The model under review builds one solid part; all positions refer to its coordinate system, in mm. A direction names the side the tool comes from. Give positions to 0.01 mm unless a question says otherwise; leave off trailing zeros. Order: outer loops, then holes, each group sorted by start corner. A loop starts at its lowest first (then second) coordinate and runs counter-clockwise, first axis right, second up. Notation, with made-up numbers: (23, -11) - (74, -11) arc R21 ccw to (74, 9) - close; hole circle Ø8 at (-38.75, -26.75). An arc over 180 degrees is marked (long way). Use CSV: the item, a comma, the result in double quotes.
```python
from build123d import *

# Parameters (mm, degrees)
F1_DEPTH    = 8
F2_R        = 1.5
F3_DEPTH    = 7.001
F4_T4_DEPTH = 8
F4_S5_R     = 1.5
F4_T6_DEPTH = 6
F5_R        = 1
F6_R        = 1
F7_R        = 3
F8_DEPTH    = 3


# Not quite as in the source:
# - a fillet or chamfer that OpenCascade refuses, or shapes differently, is made with other operations: its cross-section is extruded or revolved along the edge and cut away or added


with BuildPart() as f1:
    # F0 (on Front) → F1 (new body)
    with BuildSketch(Plane.XZ):
        Polygon((5.1, 5.1), (5.1, -5.1), (-5.1, -5.1), (-5.1, 5.1), (-5.1, 8.1), (-5.1, 17.1), (-8.1, 17.1), (-8.1, 8.1), (-8.1, -8.1), (8.1, -8.1), (8.1, 8.1), (-1.1, 8.1), (-1.1, 17.1), (-4.1, 17.1), (-4.1, 8.1), (-4.1, 5.1), align=None)
    extrude(amount=F1_DEPTH)

    # F2 (on face) → F3 (cut, through all)
    with BuildSketch(Plane.YZ.offset(-1.1)):
        with Locations((-5, 11)):
            Circle(F2_R)
    extrude(amount=-F3_DEPTH, mode=Mode.SUBTRACT)

    # F4: chamfer of 3 on 1 edges, made by hand


with BuildPart() as f4_tool2:
    # F4_s3 → F4_t4 (new body)
    with BuildSketch(Plane.XZ):
        Polygon((1.9, 8.1), (-1.1, 11.1), (-1.1, 8.1), align=None)
    extrude(amount=F4_T4_DEPTH)

    # F4_s5 → F4_t6 (cut, symmetric)
    with BuildSketch(Plane.YZ.offset(0.4)):
        with Locations((-5, 11)):
            Circle(F4_S5_R)
    extrude(amount=F4_T6_DEPTH, both=True, mode=Mode.SUBTRACT)


with BuildPart() as f1_1:
    add(f1.part)

    # F4_t1: union F4_tool2
    add(f4_tool2.part)

    # F5
    f5_edges = [f1_1.edges().sort_by_distance(p)[0] for p in [
        (8.1, -4, -8.1),
        (8.1, -4, 8.1),
        (8.1, 0, 0),
        (8.1, -8, 0),
        (-8.1, -4, -8.1),
        (0, 0, -8.1),
        (0, -8, -8.1),
        (-8.1, -4, 17.1),
        (-8.1, 0, 4.5),
        (-8.1, -8, 4.5),
        (-1.1, -4, 17.1),
        (-1.1, 0, 14.1),
        (-1.1, -8, 14.1),
    ]]
    fillet(f5_edges, radius=F5_R)

    # F6
    f6_edges = [f1_1.edges().sort_by_distance(p)[0] for p in [
        (0.4, 0, 9.6),
        (0.4, -8, 9.6),
    ]]
    fillet(f6_edges, radius=F6_R)

    # F7 (on face) → F8 (cut)
    with BuildSketch(Plane.YZ.offset(-1.1)):
        with Locations((-5, 11)):
            Circle(F7_R)
    extrude(amount=F8_DEPTH, mode=Mode.SUBTRACT)


solid = f1_1.part
```
Item 1: Mouldability with a two-part tool opening along X and no side actions: class faces 1 (the face through (7.799, -0.285, 0.606)), 2 (the face through (-5.1, -4, 6)), 3 (the face through (-6.6, -6.2, 10.1)) as pulls with the +X half, pulls with the -X half, needs draft (parallel to the pull), parting line crosses it, or undercut.
Results list:
face 1,"pulls with the +X half"
face 2,"undercut"
face 3,"needs draft"
Item 2: Wall thickness on L1, parallel to Z at x = -2.6, y = -5; L2, parallel to Y at x = -2.6, z = 11; L3, parallel to X at y = -5.5, z = -2.5: over which ranges is each line inside the solid? List them lowest first.
Results list:
L1,"z = -8.1 to -5.1, 5.1 to 9.5, 12.5 to 17.1"
L2,"y = -8 to -6.5, -3.5 to 0"
L3,"x = -8.1 to -5.1, 5.1 to 8.1"
Item 3: Take a section at B-B, the plane z = 14.25. Give the boundary of the cut face in (x, y).
Results list:
outline,"(-8.1, -7) arc R1 ccw to (-7.1, -8) - (-5.1, -8) - (-5.1, 0) - (-7.1, 0) arc R1 ccw to (-8.1, -1) - close; (-4.1, -8) - (-2.1, -8) arc R1 ccw to (-1.1, -7) - (-1.1, -1) arc R1 ccw to (-2.1, 0) - (-4.1, 0) - close"
Item 4: Take a section at C-C, the plane y = -5. Give the boundary of the cut face in (x, z), and give its area (3 significant figures).
Results list:
outline,"(-8.1, -7.1) arc R1 ccw to (-7.1, -8.1) - (7.1, -8.1) arc R1 ccw to (8.1, -7.1) - (8.1, 7.1) arc R1 ccw to (7.1, 8.1) - (1.9, 8.1) - (1.9, 8) - (-1.1, 8) - (-1.1, 9.5) - (-4.1, 9.5) - (-4.1, 5.1) - (5.1, 5.1) - (5.1, -5.1) - (-5.1, -5.1) - (-5.1, 9.5) - (-8.1, 9.5) - close; (-8.1, 12.5) - (-5.1, 12.5) - (-5.1, 17.1) - (-7.1, 17.1) arc R1 ccw to (-8.1, 16.1) - close; (-4.1, 12.5) - (-1.1, 12.5) - (-1.1, 16.1) arc R1 ccw to (-2.1, 17.1) - (-4.1, 17.1) - close"
area,"190 mm2"
Item 5: Take a section at A-A, the plane x = 4.25. Give the boundary of the cut face in (y, z), and give its area (3 significant figures).
Results list:
outline,"(-8, -7.1) arc R1 ccw to (-7, -8.1) - (-1, -8.1) arc R1 ccw to (0, -7.1) - (0, -5.1) - (-8, -5.1) - close; (-8, 5.1) - (0, 5.1) - (0, 8.1) - (-8, 8.1) - close"
area,"47.6 mm2"
Item 6: Tool access review of faces 4 (the face through (5.1, -4, 0)), 5 (the face through (-1.385, -7.699, 13.938)), 6 (the face through (-8.1, -4, 5)): name each direction out of +Z, -Z, +X, -X, +Y, -Y from which nothing blocks a thin tool from reaching the whole face with its end or side.
Results list:
face 4,"+Y, -Y"
face 5,"+Z, +X, -Y"
face 6,"+Z, -Z, -X, +Y, -Y"
Item 7: Take a section at D-D, the plane x = -5.5. Give the boundary of the cut face in (y, z), and give its area (3 significant figures).
Results list:
outline,"(-8, -7.1) arc R1 ccw to (-7, -8.1) - (-1, -8.1) arc R1 ccw to (0, -7.1) - (0, 17.1) - (-8, 17.1) - close; hole circle Ø3 at (-5, 11)"
area,"194 mm2"
